```python
from build123d import *

# Parameters (mm, degrees)
SKETCH1_W               = 240
SKETCH1_H               = 45
SKETCH1_R               = 1.5
SKETCH1_W_2             = 5
SKETCH1_H_2             = 10
BOSS_EXTRUDE1_DEPTH     = 5
ESQUISSE1_W             = 210
ESQUISSE1_H             = 25
ENL_V_MAT_EXTRU_1_DEPTH = 10
CONG_1_R                = 5


with BuildPart() as part:
    # Sketch1 → Boss-Extrude1 (new body)
    with BuildSketch(Plane.XY):
        with Locations((34.186746988, 0)):
            Rectangle(SKETCH1_W, SKETCH1_H)
        with Locations((-78.313253012, 0)):
            Circle(SKETCH1_R, mode=Mode.SUBTRACT)
        with Locations(Location((146.686746988, 0, 0), (0, 0, 180))):
            Circle(SKETCH1_R, mode=Mode.SUBTRACT)
        with Locations((-78.313253012, -15)):
            Rectangle(SKETCH1_W_2, SKETCH1_H_2, mode=Mode.SUBTRACT)
        with Locations((-78.313253012, 15)):
            Rectangle(SKETCH1_W_2, SKETCH1_H_2, mode=Mode.SUBTRACT)
        with Locations((146.686746988, -15)):
            Rectangle(SKETCH1_W_2, SKETCH1_H_2, mode=Mode.SUBTRACT)
        with Locations((146.686746988, 15)):
            Rectangle(SKETCH1_W_2, SKETCH1_H_2, mode=Mode.SUBTRACT)
    extrude(amount=BOSS_EXTRUDE1_DEPTH)

    # Esquisse1 → Enlèv. mat.-Extru.1 (cut)
    with BuildSketch(Plane.XY.offset(5)):
        with Locations((34.186746988, 0)):
            Rectangle(ESQUISSE1_W, ESQUISSE1_H)
    extrude(amount=-ENL_V_MAT_EXTRU_1_DEPTH, mode=Mode.SUBTRACT)

    # Congé1
    cong_1_edges = [part.edges().sort_by_distance(p)[0] for p in [
        (-85.813253012, 22.5, 2.5),
        (154.186746988, 22.5, 2.5),
        (154.186746988, -22.5, 2.5),
        (-85.813253012, -22.5, 2.5),
        (-70.813253012, -12.5, 2.5),
        (-70.813253012, 12.5, 2.5),
        (139.186746988, 12.5, 2.5),
        (139.186746988, -12.5, 2.5),
    ]]
    fillet(cong_1_edges, radius=CONG_1_R)


solid = part.part
```
Source: CAD feature listing. Evaluate the final solid. Frame: model axes, mm. A direction names the side the tool comes from. Give positions to 0.01 mm unless a question says otherwise; leave off trailing zeros. Loops run counter-clockwise (first coordinate to the right, second up) from the corner with the lowest first, then second, coordinate; pieces in that order, holes last. Notation, with made-up numbers: M 59,20.25 L 115,20.25 A26 ccw 115,50.25 Z; hole C 66.5,43.25 d2. An arc over 180 degrees is marked long. Put each result on its own line as item: value.
Q1. Section A-A (x = 83). Return the cut outline in (y, z), and give its area (3 significant figures).
Response values:
outline: M -22.5,0 L -12.5,0 L -12.5,5 L -22.5,5 Z; M 12.5,0 L 22.5,0 L 22.5,5 L 12.5,5 Z
area: 100 mm²
Q2. Pin query (flat end, axial travel): P1, Ø1.8, axis at x = 146.69, y = 0, coming from the -Z side. Return the tip coordinate at first contact, or that it passes through.
Response values:
P1: passes through
Q3. Section B-B (z = 3.7). Count the separate pieces of the cut face and the enclosed holes in it, and give its area (3 significant figures).
Response values:
separate pieces: 1
enclosed holes: 7
area: 5,340 mm²
Q4. Line query: probe 1 along X at (y, z) = (-14, 2.35); probe 2 along Y at (x, z) = (42.5, 0.35); probe 3 along X at (y, z) = (19, 0.55). Output: solid intervals per line, ascending. Write a range as [from, to].
Response values:
probe 1: x = [-85.81, -80.81], [-75.81, 144.19], [149.19, 154.19]
probe 2: y = [-22.5, -12.5], [12.5, 22.5]
probe 3: x = [-85.58, -80.81], [-75.81, 144.19], [149.19, 153.96]
Q5. Reachability of faces 5 (the cylindrical face through (-84.387, 20.996, 2.535)), 6 (the flat face through (-78, -10, 2)) from +Z, -Z, +X, -X, +Y, -Y: full face, straight path, thin tool, end or side. Return the list, or none.
Response values:
face 5: +Z, -Z, -X, +Y
face 6: +Z, -Z
Q6. Mould query, pull axis Y, two halves, no side actions, for faces 1 (the flat face through (33, 15, 0)), 2 (the cylindrical face through (-84.387, -20.996, 2.535)), 3 (the flat face through (33, 22.5, 2)), 4 (the flat face through (144.187, -15, 2)). Classes: released by +Y, released by -Y, zero draft, split by the parting line, or undercut.
Response values:
face 1: zero draft
face 2: released by -Y
face 3: released by +Y
face 4: undercut
